Work out the finished part from the listing and answer in its coordinate system (mm). Coordinates: 2 decimals unless noted, no trailing zeros. Write each loop counter-clockwise with the first axis right and the second up, starting at its lowest first coordinate (ties: lowest second). Pieces come first, ordered by that corner, then holes. Notation, with made-up numbers: (64, 44.5) - (107, 44.5) arc R13 ccw to (107, 57.5) - close; hole circle Ø8 at (-12.75, 37). An arc over 180 degrees is marked (long way). Use a Markdown table: item, result. Add a question column.
(1) The part is cut by section B-B, the plane x = -317. Give the vertices of the cut face in (y, z) (3 decimals), then the cut area to 3 significant figures.
(2) The part is cut by section A-A, the plane y = 224.79. Give the vertices of the cut face in (x, z) (3 decimals).
(3) The part is cut by section C-C, the plane z = 1.55. State how many separate pieces and enclosed holes the cut face has, then the cut area to 3 significant figures.
(4) Find the intervals of material crossed by line 1 (Y direction, x = -280, z = 2.05); line 2 (Y direction, x = -317, z = 2.1); line 3 (Y direction, x = -350, z = 0.9), in increasing order. Write a range as from..to.
from build123d import *

# Parameters (mm, degrees)
BOSS_EXTRUDE1_DEPTH = 3.175
SKETCH3_R           = 2.5
CUT_EXTRUDE2_DEPTH  = 4.175
CUT_EXTRUDE3_DEPTH  = 4.175


with BuildPart() as part:
    # Sketch1 → Boss-Extrude1 (new body)
    with BuildSketch(Plane.XY):
        with BuildLine():
            Line((-367.50625, 254), (-240.50625, 254))
            ThreePointArc((-240.50625, 254), (-236.016121939, 252.140128061), (-234.15625, 247.65))
            Line((-234.15625, 247.65), (-234.15625, 69.85))
            ThreePointArc((-234.15625, 69.85), (-236.016121939, 65.359871939), (-240.50625, 63.5))
            Line((-240.50625, 63.5), (-367.50625, 63.5))
            ThreePointArc((-367.50625, 63.5), (-371.996378061, 65.359871939), (-373.85625, 69.85))
            Line((-373.85625, 69.85), (-373.85625, 247.65))
            ThreePointArc((-373.85625, 247.65), (-371.996378061, 252.140128061), (-367.50625, 254))
        make_face()
    extrude(amount=BOSS_EXTRUDE1_DEPTH)

    # Sketch3 → Cut-Extrude2 (cut, through all)
    with BuildSketch(Plane.XY.offset(3.175)):
        with Locations((-367.50625, 247.65)):
            Circle(SKETCH3_R)
        with Locations((-367.50625, 69.85)):
            Circle(SKETCH3_R)
        with Locations((-354.80625, 247.65)):
            Circle(SKETCH3_R)
        with Locations((-354.80625, 69.85)):
            Circle(SKETCH3_R)
        with Locations((-342.10625, 247.65)):
            Circle(SKETCH3_R)
        with Locations((-342.10625, 69.85)):
            Circle(SKETCH3_R)
        with Locations((-329.40625, 247.65)):
            Circle(SKETCH3_R)
        with Locations((-329.40625, 69.85)):
            Circle(SKETCH3_R)
        with Locations((-316.70625, 247.65)):
            Circle(SKETCH3_R)
        with Locations((-316.70625, 69.85)):
            Circle(SKETCH3_R)
        with Locations((-304.00625, 247.65)):
            Circle(SKETCH3_R)
        with Locations((-304.00625, 69.85)):
            Circle(SKETCH3_R)
        with Locations((-291.30625, 247.65)):
            Circle(SKETCH3_R)
        with Locations((-291.30625, 69.85)):
            Circle(SKETCH3_R)
        with Locations((-278.60625, 247.65)):
            Circle(SKETCH3_R)
        with Locations((-278.60625, 69.85)):
            Circle(SKETCH3_R)
        with Locations((-265.90625, 247.65)):
            Circle(SKETCH3_R)
        with Locations((-265.90625, 69.85)):
            Circle(SKETCH3_R)
        with Locations((-253.20625, 247.65)):
            Circle(SKETCH3_R)
        with Locations((-253.20625, 69.85)):
            Circle(SKETCH3_R)
        with Locations((-240.50625, 247.65)):
            Circle(SKETCH3_R)
        with Locations((-240.50625, 69.85)):
            Circle(SKETCH3_R)
    extrude(amount=-CUT_EXTRUDE2_DEPTH, mode=Mode.SUBTRACT)

    # Sketch4 → Cut-Extrude3 (cut, through all)
    with BuildSketch(Plane.XY.offset(3.175)):
        with BuildLine():
            Line((-357.98125, 234.315), (-351.63125, 234.315))
            ThreePointArc((-351.63125, 234.315), (-348.45625, 237.49), (-351.63125, 240.665))
            Line((-351.63125, 240.665), (-357.98125, 240.665))
            ThreePointArc((-357.98125, 240.665), (-361.15625, 237.49), (-357.98125, 234.315))
        make_face()
        with BuildLine():
            Line((-357.98125, 221.615), (-351.63125, 221.615))
            ThreePointArc((-351.63125, 221.615), (-348.45625, 224.79), (-351.63125, 227.965))
            Line((-351.63125, 227.965), (-357.98125, 227.965))
            ThreePointArc((-357.98125, 227.965), (-361.15625, 224.79), (-357.98125, 221.615))
        make_face()
        with BuildLine():
            ThreePointArc((-256.38125, 221.615), (-259.55625, 224.79), (-256.38125, 227.965))
            Line((-256.38125, 227.965), (-250.03125, 227.965))
            ThreePointArc((-250.03125, 227.965), (-246.85625, 224.79), (-250.03125, 221.615))
            Line((-250.03125, 221.615), (-256.38125, 221.615))
        make_face()
        with BuildLine():
            ThreePointArc((-256.38125, 234.315), (-259.55625, 237.49), (-256.38125, 240.665))
            Line((-256.38125, 240.665), (-250.03125, 240.665))
            ThreePointArc((-250.03125, 240.665), (-246.85625, 237.49), (-250.03125, 234.315))
            Line((-250.03125, 234.315), (-256.38125, 234.315))
        make_face()
        with BuildLine():
            ThreePointArc((-351.63125, 95.885), (-348.45625, 92.71), (-351.63125, 89.535))
            Line((-351.63125, 89.535), (-357.98125, 89.535))
            ThreePointArc((-357.98125, 89.535), (-361.15625, 92.71), (-357.98125, 95.885))
            Line((-357.98125, 95.885), (-351.63125, 95.885))
        make_face()
        with BuildLine():
            ThreePointArc((-351.63125, 83.185), (-348.45625, 80.01), (-351.63125, 76.835))
            Line((-351.63125, 76.835), (-357.98125, 76.835))
            ThreePointArc((-357.98125, 76.835), (-361.15625, 80.01), (-357.98125, 83.185))
            Line((-357.98125, 83.185), (-351.63125, 83.185))
        make_face()
        with BuildLine():
            Line((-250.03125, 95.885), (-256.38125, 95.885))
            ThreePointArc((-256.38125, 95.885), (-259.55625, 92.71), (-256.38125, 89.535))
            Line((-256.38125, 89.535), (-250.03125, 89.535))
            ThreePointArc((-250.03125, 89.535), (-246.85625, 92.71), (-250.03125, 95.885))
        make_face()
        with BuildLine():
            Line((-250.03125, 83.185), (-256.38125, 83.185))
            ThreePointArc((-256.38125, 83.185), (-259.55625, 80.01), (-256.38125, 76.835))
            Line((-256.38125, 76.835), (-250.03125, 76.835))
            ThreePointArc((-250.03125, 76.835), (-246.85625, 80.01), (-250.03125, 83.185))
        make_face()
    extrude(amount=-CUT_EXTRUDE3_DEPTH, mode=Mode.SUBTRACT)


solid = part.part
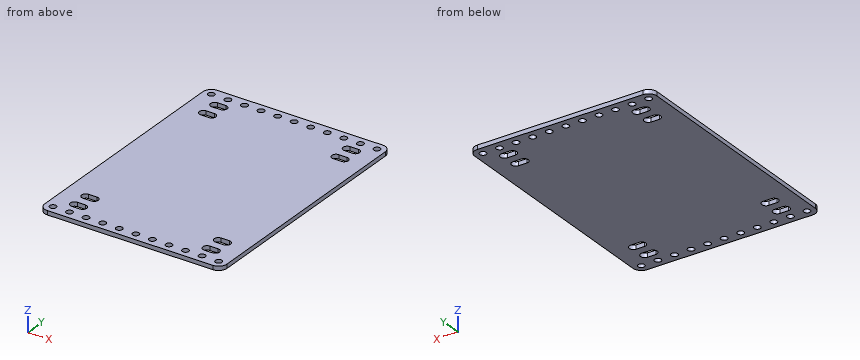
Model answer:
| question | item | result |
|---|---|---|
| 1 | outline | (63.5, 0) - (67.367, 0) - (67.367, 3.175) - (63.5, 3.175) - close; (72.333, 0) - (245.167, 0) - (245.167, 3.175) - (72.333, 3.175) - close; (250.133, 0) - (254, 0) - (254, 3.175) - (250.133, 3.175) - close |
| 1 | area | 573 mm^2 |
| 2 | outline | (-373.856, 0) - (-361.156, 0) - (-361.156, 3.175) - (-373.856, 3.175) - close; (-348.456, 0) - (-259.556, 0) - (-259.556, 3.175) - (-348.456, 3.175) - close; (-246.856, 0) - (-234.156, 0) - (-234.156, 3.175) - (-246.856, 3.175) - close |
| 3 | separate pieces | 1 |
| 3 | enclosed holes | 30 |
| 3 | area | 25,600 mm^2 |
| 4 | line 1 | 63.5..67.77, 71.93..245.57, 249.73..254 |
| 4 | line 2 | 63.5..67.37, 72.33..245.17, 250.13..254 |
| 4 | line 3 | 63.5..77.29, 82.73..89.99, 95.43..222.07, 227.51..234.77, 240.21..254 |
